from build123d import *

# Parameters (mm, degrees)
SALIENTE_EXTRUIR1_DEPTH   = 0.1
SALIENTE_EXTRUIR1_2_DEPTH = 0.1
CROQUIS7_R                = 2.9
SALIENTE_EXTRUIR2_DEPTH   = 1


with BuildPart() as part:
    # Croquis1 → Saliente-Extruir1 (new, symmetric)
    with BuildSketch(Plane.XY):
        with BuildLine():
            Line((2.141229394, -3.596955899), (1.261229394, -3.596955899))
            Line((1.261229394, -3.596955899), (1.261229394, -2.896955899))
            Line((1.261229394, -2.896955899), (1.267504118, -2.896955899))
            ThreePointArc((1.267504118, -2.896955899), (1.465494017, -2.814945798), (1.547504118, -2.616955899))
            Line((1.547504118, -2.616955899), (1.547504118, 0.274513326))
            Line((1.547504118, 0.274513326), (1.547504118, 1.461848277))
            Line((1.547504118, 1.461848277), (0.641229394, 1.974513326))
            Line((0.641229394, 1.974513326), (0.641229394, 4.774513326))
            Line((0.641229394, 4.774513326), (2.841229394, 4.774513326))
            Line((2.841229394, 4.774513326), (2.841229394, 1.461848277))
            Line((2.841229394, 1.461848277), (2.641229394, 1.461848277))
            Line((2.641229394, 1.461848277), (2.641229394, 0.274513326))
            Line((2.641229394, 0.274513326), (2.641229394, -24.225486674))
            Line((2.641229394, -24.225486674), (2.141229394, -24.225486674))
            Line((2.141229394, -24.225486674), (2.141229394, -3.596955899))
        make_face()
    extrude(amount=SALIENTE_EXTRUIR1_DEPTH, both=True)



with BuildPart() as body_2:
    # Croquis1 → Saliente-Extruir1 2 (new, symmetric)
    with BuildSketch(Plane.XY):
        with BuildLine():
            Line((-0.398770606, 0.274513326), (-0.398770606, -2.896955899))
            Line((-0.398770606, -2.896955899), (-0.498770606, -2.896955899))
            ThreePointArc((-0.498770606, -2.896955899), (-0.604836624, -2.940889882), (-0.648770606, -3.046955899))
            Line((-0.648770606, -3.046955899), (-0.648770606, -3.446955899))
            ThreePointArc((-0.648770606, -3.446955899), (-0.604836624, -3.553021917), (-0.498770606, -3.596955899))
            Line((-0.498770606, -3.596955899), (-0.398770606, -3.596955899))
            Line((-0.398770606, -3.596955899), (-0.398770606, -25.725486674))
            Line((-0.398770606, -25.725486674), (0.101229394, -25.725486674))
            Line((0.101229394, -25.725486674), (0.101229394, -3.596955899))
            Line((0.101229394, -3.596955899), (0.201229394, -3.596955899))
            ThreePointArc((0.201229394, -3.596955899), (0.307295411, -3.553021917), (0.351229394, -3.446955899))
            Line((0.351229394, -3.446955899), (0.351229394, -3.046955899))
            ThreePointArc((0.351229394, -3.046955899), (0.307295411, -2.940889882), (0.201229394, -2.896955899))
            Line((0.201229394, -2.896955899), (0.101229394, -2.896955899))
            Line((0.101229394, -2.896955899), (0.101229394, 0.274513326))
            Line((0.101229394, 0.274513326), (0.101229394, 4.774513326))
            Line((0.101229394, 4.774513326), (-0.398770606, 4.774513326))
            Line((-0.398770606, 4.774513326), (-0.398770606, 2.056181546))
            Line((-0.398770606, 2.056181546), (-0.898770606, 0.945997951))
            Line((-0.898770606, 0.945997951), (-0.898770606, 0.274513326))
            Line((-0.898770606, 0.274513326), (-0.398770606, 0.274513326))
        make_face()
    extrude(amount=SALIENTE_EXTRUIR1_2_DEPTH, both=True)


with BuildPart() as part_1:
    add(part.part)

    add(body_2.part)  # Saliente-Extruir2 merges body 2
    # Croquis7 → Saliente-Extruir2 (add)
    with BuildSketch(Plane(origin=(0, 0.274513326, 0), x_dir=(-1, 0, 0), z_dir=(0, -1, 0))):
        with Locations(Location((-1.121229394, 0, 0), (0, 0, 90))):
            Circle(CROQUIS7_R)
    extrude(amount=-SALIENTE_EXTRUIR2_DEPTH)

    # Croquis9 → Revolución2 (revolve)
    with BuildSketch(Plane.XY, mode=Mode.PRIVATE) as revoluci_n2_sk:
        with BuildLine():
            Line((-1.370805616, 1.274513326), (-1.370805616, 6.27937105))
            ThreePointArc((-1.370805616, 6.27937105), (-0.641386379, 8.044319707), (1.121229394, 8.779358362))
            Line((1.121229394, 8.779358362), (1.121229394, 8.681444496))
            Line((1.121229394, 8.681444496), (1.021229394, 8.676941396))
            ThreePointArc((1.021229394, 8.676941396), (-0.605613383, 7.937816712), (-1.270805616, 6.27937105))
            Line((-1.270805616, 6.27937105), (-1.270805616, 1.274513326))
            Line((-1.270805616, 1.274513326), (-1.370805616, 1.274513326))
        make_face()
    revolve(revoluci_n2_sk.sketch.rotate(Axis((1.121229394, 8.681444496, 0), (0, -1, 0)), 270), axis=Axis((1.121229394, 8.681444496, 0), (0, -1, 0)))


solid = part_1.part
CAD build for the part. Positions are in the model's coordinates, mm. A direction names the side the tool comes from. Round coordinates to 2 decimals unless told otherwise and drop trailing zeros. Write each loop counter-clockwise with the first axis right and the second up, starting at its lowest first coordinate (ties: lowest second). Pieces come first, ordered by that corner, then holes. Notation, with made-up numbers: (2, 16.5) -> (49, 16.5) arc R12 cw to (49, 24.5) -> close; hole circle Ø7 at (81, 17). An arc over 180 degrees is marked (long way). Answer as a JSON object with one key per item and string values.
(1) Band-saw the part on A-A, the plane y = -9. List the corners of the cut face in (x, z), then the cut area to 3 significant figures.
Reported:
{"outline": "(-0.4, -0.1) -> (0.1, -0.1) -> (0.1, 0.1) -> (-0.4, 0.1) -> close; (2.14, -0.1) -> (2.64, -0.1) -> (2.64, 0.1) -> (2.14, 0.1) -> close", "area": "0.200 mm^2"}
(2) Which spindle directions (+Z, -Z, +X, -X, +Y, -Y) get a long thin tool onto all of the face, cutting with end or side? Do faces 1 (the face through (-0.2, -12.5, -0.1)), 2 (the face through (-0.1, 3, 0.1)), 3 (the face through (2.4, -9.1, 0.1)). Say none if no direction does.
Reported:
{"face 1": "-Z, +X, -X, -Y", "face 2": "none", "face 3": "+Z, +X, -X, -Y"}
(3) Probe probe 1 along Y at (x, z) = (3.85, -0.8); probe 2 along Y at (x, z) = (-0.85, 0.55); probe 3 along Y at (x, z) = (2.85, 0.6). List the from-to ranges inside material, lowest first. Write a range as [from, to].
Reported:
{"probe 1": "y = [0.27, 1.27]", "probe 2": "y = [0.27, 1.27], [7.52, 7.7]", "probe 3": "y = [0.27, 1.27], [7.82, 7.97]"}
(4) Pin check, flat tips, straight feed: P1, Ø2, axis at x = 1, y = -13, coming from the +Z side; P2, Ø2.5, axis at x = 2, y = 3, coming from the -Z side; P3, Ø0.8, axis at x = 0, y = -11, coming from the -Z side; P4, Ø3, axis at x = 1, z = -0.5, coming from the +Y side. Stop position of each tip, or through.
Reported:
{"P1": "stops at z = 0.1", "P2": "stops at z = -2.49", "P3": "stops at z = -0.1", "P4": "stops at y = 8.78"}
(5) Two-plate mould, pull along Z, no slides. Class faces 4 (the face through (-0.1, 3, -0.1)), 5 (the face through (-0.2, -12.5, 0.1)), 6 (the face through (1.2, 0.8, 2.9)): +Z half, -Z half, draft (parallel to the pull), parting line (faces both ways), or undercut.
Reported:
{"face 4": "undercut", "face 5": "+Z half", "face 6": "parting line"}
